Can you work these out from the drawing? Everything is in mm from the part's minimum corner. Round coordinates to 2 decimals unless told otherwise and drop trailing zeros. Loops run counter-clockwise (first coordinate to the right, second up) from the corner with the lowest first, then second, coordinate; pieces in that order, holes last. Notation, with made-up numbers: (1.5, 84) -> (17.5, 84) arc R31 cw to (17.5, 117) -> close; hole circle Ø10 at (40.5, -29.5). An arc over 180 degrees is marked (long way). One line per item, written item: value.
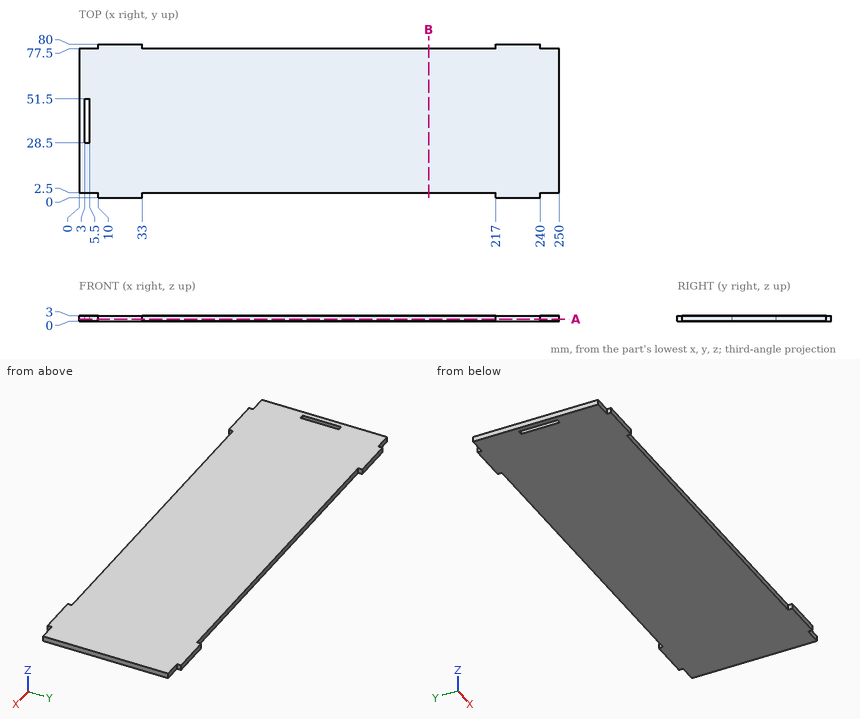
(1) I'm going to push flat-ended pins straight in: pin 1 Ø1.2 at (y, z) = (1.5, 1) entering from +X; pin 2 Ø0.9 at (x, z) = (244.5, 1) entering from -Y; pin 3 Ø1.2 at (x, z) = (4.5, 2) entering from +Y. Where does each tip first touch, or does it pass through?
Recorded:
pin 1: x = 240
pin 2: y = 2.5
pin 3: y = 77.5
(2) If we section it at A-A, the plane z = 1.2: Please give me the cut outline in (x, y), then the cut area to 3 significant figures.
Recorded:
outline: (0, 2.5) -> (10, 2.5) -> (10, 0) -> (33, 0) -> (33, 2.5) -> (217, 2.5) -> (217, 0) -> (240, 0) -> (240, 2.5) -> (250, 2.5) -> (250, 77.5) -> (240, 77.5) -> (240, 80) -> (217, 80) -> (217, 77.5) -> (33, 77.5) -> (33, 80) -> (10, 80) -> (10, 77.5) -> (0, 77.5) -> close; hole (3, 28.5) -> (5.5, 28.5) -> (5.5, 51.5) -> (3, 51.5) -> close
area: 18,900 mm²
(3) If I drill on L1, parallel to X at y = 38, z = 1.2; L2, parallel to Y at x = 94.5, z = 0.15, over which ranges is the centre line in solid material (lowest first)?
Recorded:
L1: 0 to 3, 5.5 to 250
L2: 2.5 to 77.5
(4) If we section it at B-B, the plane x = 182: Please give me the cut outline in (y, z), then the cut area to 3 significant figures.
Recorded:
outline: (2.5, 0) -> (77.5, 0) -> (77.5, 3) -> (2.5, 3) -> close
area: 225 mm²
